Here's the drawing with two shaded views (mm, measured from the low corner). I have some questions. Round coordinates to 2 decimals unless told otherwise and drop trailing zeros. Loops run counter-clockwise (first coordinate to the right, second up) from the corner with the lowest first, then second, coordinate; pieces in that order, holes last. Notation, with made-up numbers: (88.5, 3.5) -> (140.5, 3.5) arc R16 ccw to (140.5, 30.5) -> close; hole circle Ø9 at (15.5, 1). An arc over 180 degrees is marked (long way). Write item = value, one per line.
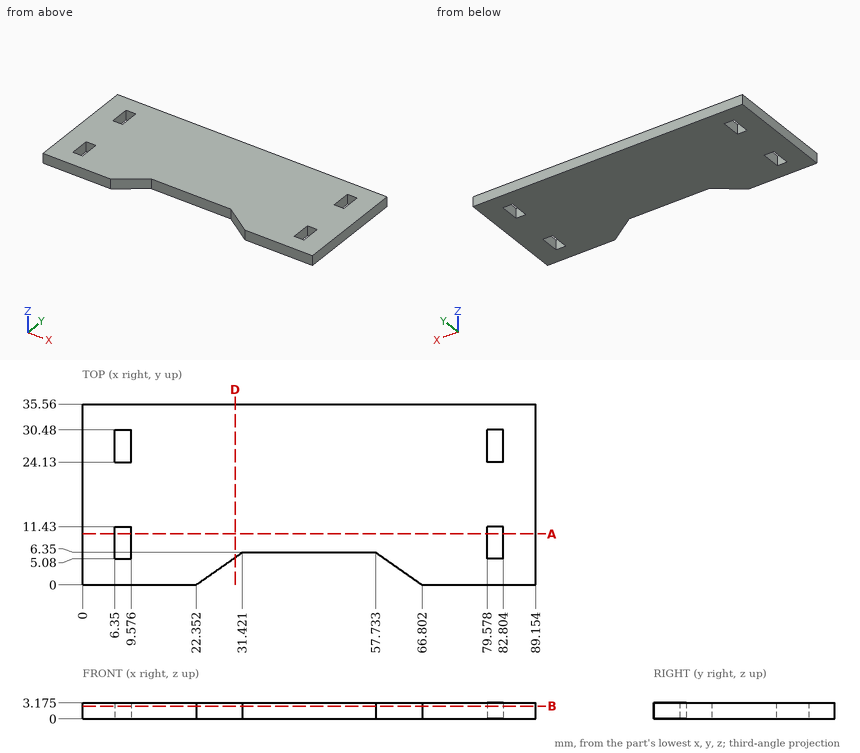
1. Suppose I cut it at D-D, the plane x = 30. List the corners of the cut face in (y, z) for me (1 decimal), and give its area (3 significant figures).
Entries:
outline = (5.4, 0) -> (35.6, 0) -> (35.6, 3.2) -> (5.4, 3.2) -> close
area = 95.9 mm²
2. Suppose I cut it at A-A, the plane y = 10. Count the separate pieces of the cut face and the enclosed holes in it.
Entries:
separate_pieces = 3
enclosed_holes = 0
3. I'm going to push a flat-ended pin straight in: pin 1 (1.6 mm diameter, centred on y = 8.5, z = 1.5, fed in from -X). Where does the tip first touch, or does it pass through?
Entries:
pin_1 = 0
4. Suppose I cut it at B-B, the plane z = 2.5. List the corners of the cut face in (x, y) for me.
Entries:
outline = (0, 0) -> (22.35, 0) -> (31.42, 6.35) -> (57.73, 6.35) -> (66.8, 0) -> (89.15, 0) -> (89.15, 35.56) -> (0, 35.56) -> close; hole (6.35, 5.08) -> (9.58, 5.08) -> (9.58, 11.43) -> (6.35, 11.43) -> close; hole (6.35, 24.13) -> (9.58, 24.13) -> (9.58, 30.48) -> (6.35, 30.48) -> close; hole (79.58, 5.08) -> (82.8, 5.08) -> (82.8, 11.43) -> (79.58, 11.43) -> close; hole (79.58, 24.13) -> (82.8, 24.13) -> (82.8, 30.48) -> (79.58, 30.48) -> close
5. I need wall thicknesses on line 1 (X direction, y = 25, z = 2); line 2 (Y direction, x = 34.5, z = 0.4); line 3 (Y direction, x = 27.5, z = 0.7) (1 decimal). Which ranges of each line are inside material? Lowest first, please. Write a range as [from, to].
Entries:
line_1 = [0, 6.35], [9.58, 79.58], [82.8, 89.15]
line_2 = [6.35, 35.56]
line_3 = [3.6, 35.6]
